from build123d import *

# Parameters (mm, degrees)
SKETCH_1_W          = 43
SKETCH_1_H          = 43
EXTRUDE_1_DEPTH     = 32
SKETCH_5_W          = 10.30081486
SKETCH_5_H          = 4.860243631
CUT_EXTRUDE_1_DEPTH = 18
SKETCH_6_R          = 20.5
EXTRUDE_2_DEPTH     = 66
SKETCH_7_R          = 2
CUT_EXTRUDE_2_DEPTH = 30


with BuildPart() as part:
    # 草图1 → 凸台-拉伸1 (new body)
    with BuildSketch(Plane.XY):
        Rectangle(SKETCH_1_W, SKETCH_1_H)
    extrude(amount=EXTRUDE_1_DEPTH)

    # 草图4 → 旋转1 (revolve)
    with BuildSketch(Plane(origin=(0, 0, 0), x_dir=(0, 0, -1), z_dir=(1, 0, 0))):
        Polygon((0, 0), (0, 7), (7, 7), (7, 4), (27, 4), (27, 0), align=None)
    revolve(axis=Axis((0, 0, -27), (0, 0, 1)))

    # 草图5 → 切除-拉伸1 (cut)
    with BuildSketch(Plane(origin=(0, 0, -27), x_dir=(-1, 0, 0), z_dir=(0, 0, -1))):
        with Locations((0.230133924, 5.430121815)):
            Rectangle(SKETCH_5_W, SKETCH_5_H)
    extrude(amount=-CUT_EXTRUDE_1_DEPTH, mode=Mode.SUBTRACT)

    # 草图6 → 凸台-拉伸2 (add)
    with BuildSketch(Plane.XY.offset(32)):
        Circle(SKETCH_6_R)
    extrude(amount=EXTRUDE_2_DEPTH)

    # 草图7 → 切除-拉伸2 (cut)
    with BuildSketch(Plane(origin=(0, 0, 0), x_dir=(-1, 0, 0), z_dir=(0, 0, -1))):
        with Locations((-18, 18)):
            Circle(SKETCH_7_R)
        with Locations((18, 18)):
            Circle(SKETCH_7_R)
        with Locations((18, -18)):
            Circle(SKETCH_7_R)
        with Locations((-18, -18)):
            Circle(SKETCH_7_R)
    extrude(amount=-CUT_EXTRUDE_2_DEPTH, mode=Mode.SUBTRACT)


solid = part.part
Build history of the part. All positions in model axes, mm. A direction names the side the tool comes from. Round coordinates to 2 decimals unless told otherwise and drop trailing zeros. Write each loop counter-clockwise with the first axis right and the second up, starting at its lowest first coordinate (ties: lowest second). Pieces come first, ordered by that corner, then holes. Notation, with made-up numbers: M -30,-25 L 11,-25 A15 cw 11,-15 Z; hole C -33.5,20 d5. An arc over 180 degrees is marked long. Answer as a JSON object with one key per item and string values. Group by question number.
(1) Cut at A-A (x = 0). Give the cut face in (y, z), and give its area (3 significant figures).
(2) Flat gauge pins, fed straight in: pin 1 (3.5 mm diameter, centred on x = 18, y = -18, fed in from -Z); pin 2 (6 mm diameter, centred on y = 10.5, z = 64.5, fed in from +X); pin 3 (3 mm diameter, centred on x = 19, y = 17.5, fed in from -Z); pin 4 (5 mm diameter, centred on x = -14, y = -15, fed in from +Z). Where does each tip first touch, or does it go through?
(3) Cut at B-B (y = -8.5). Give the cut face in (x, z), and give its area (3 significant figures).
(4) Cut at C-C (z = -5.5). Give the cut face in (x, y).
(5) Which spindle directions (+Z, -Z, +X, -X, +Y, -Y) get a long thin tool onto all of the face, cutting with end or side? Do faces 4 (the flat face through (0, -21.5, 16)), 5 (the cylindrical face through (-4.444, -20.013, 64.538)), 6 (the cylindrical face through (0, -4, -17)). Say none if no direction does.
(6) Drill centre lines: L1, parallel to Y at x = -18, z = 23; L2, parallel to Z at x = -9.5, y = -16.5; L3, parallel to Z at x = 11, y = 18.5. Where is each one in solid material? Low to high.
(7) Mould opens along Y. For faces 1 (the cylindrical face through (-18, -16, 15)), 2 (the flat face through (1, 21, 32)), 3 (the flat face through (0, 3, -18)) say: pulls with the +Y half, pulls with the -Y half, needs draft (parallel to the pull), parting line crosses it, or undercut.
(8) Cut at D-D (x = -13.5). Give the cut face in (y, z).
Responses:
{
 "1": {"outline": "M -21.5,0 L -7,0 L -7,-7 L -4,-7 L -4,-27 L 3,-27 L 3,-9 L 4,-9 L 4,-7 L 7,-7 L 7,0 L 21.5,0 L 21.5,32 L 20.5,32 L 20.5,98 L -20.5,98 L -20.5,32 L -21.5,32 Z", "area": "4,320 mm2"},
 "2": {"pin 1": "stops at z = 30", "pin 2": "stops at x = 19.08", "pin 3": "stops at z = 0", "pin 4": "stops at z = 98"},
 "3": {"outline": "M -21.5,0 L 21.5,0 L 21.5,32 L 18.65,32 L 18.65,98 L -18.65,98 L -18.65,32 L -21.5,32 Z", "area": "3,840 mm2"},
 "4": {"outline": "C 0,0 d14"},
 "5": {"face 4": "+Z, -Z, +X, -X, -Y", "face 5": "+Z", "face 6": "-Z"},
 "6": {"L1": "y = -21.5 to -20, -16 to 16, 20 to 21.5", "L2": "z = 0 to 98", "L3": "z = 0 to 32"},
 "7": {"face 1": "undercut", "face 2": "needs draft", "face 3": "pulls with the +Y half"},
 "8": {"outline": "M -21.5,0 L 21.5,0 L 21.5,32 L 15.43,32 L 15.43,98 L -15.43,98 L -15.43,32 L -21.5,32 Z"}
}
